Read the model definition and answer for the solid it produces. Units are mm, in the model's axes. A direction names the side the tool comes from. Coordinates: 2 decimals unless noted, no trailing zeros. Loops run counter-clockwise (first coordinate to the right, second up) from the corner with the lowest first, then second, coordinate; pieces in that order, holes last. Notation, with made-up numbers: (62.5, -8) -> (67.5, -8) arc R35 cw to (67.5, 24) -> close; hole circle Ø2 at (22, 81.25). An arc over 180 degrees is marked (long way). Answer as a JSON object with one key per item and string values. Group by question number.
Q1. The part is cut by section C-C on x = -368. Write down the section's boundary in (y, z), and give its area (3 significant figures).
Q2. Each of these flat-tipped pins is pushed along its axis until it touches: P1, Ø2, axis at x = -12.5, y = 1.5, coming from the -Z side; P2, Ø6, axis at x = -262, z = 110.5, coming from the -Y side; P3, Ø12, axis at x = -310, y = -23, coming from the +Z side; P4, Ø2, axis at y = -34.5, z = 35.5, coming from the -X side. Where does it stop, or does it pass through?
Q3. The part is cut by section B-B on x = -136. Write down the section's boundary in (y, z), and give its area (3 significant figures).
Q4. Determine the mould class of faces 1 (the cylindrical face through (396.261, -12.828, -5.883)), 2 (the flat face through (321.003, -19, -14)), 3 (the flat face through (-258, -9.876, 54)) for opening direction Z: released by +Z, released by -Z, zero draft, split by the parting line, or undercut.
Q5. For faces 4 (the flat face through (-217.761, -25, 54)), 5 (the flat face through (-321.003, -14, -7)), 6 (the flat face through (-258, -40.692, 54)), determine the directions among +Z, -Z, +X, -X, +Y, -Y from which every point of the face is accessible in a straight line to the end or side of a thin tool.
Q6. Straight lines are drawn through the part: line 1 along Z through (x, y) = (313, -17.5); line 2 along X through (y, z) = (11, 110); line 3 along Y through (x, z) = (-270, -22). For each, find the intervals that lie inside material, in ascending order. Write a range as [from, to].
Q7. The part is cut by section A-A on z = 0. Write down the section's boundary in (x, y).
from build123d import *

# Parameters (mm, degrees)
F0_W      = 642.00504
F0_H      = 59.35203
F1_DEPTH  = 50.8
F2_R      = 13.138682
F3_DEPTH  = 181.356
F4_R      = 15.361359
F5_DEPTH  = 152.654
F6_W      = 78.62696
F6_H      = 30.816156
F7_DEPTH  = 48.514
F9_R      = 16.886995
F10_DEPTH = 101.6


with BuildPart() as f1:
    # F0 (on Front) → F1 (new body)
    with BuildSketch(Plane.XZ):
        Rectangle(F0_W, F0_H)
    extrude(amount=F1_DEPTH)

    # F2 (on face) → F3 (join)
    with BuildSketch(Plane(origin=(-321.00252, 0, 0), x_dir=(0, -1, 0), z_dir=(-1, 0, 0))):
        with Locations((26.228841, 0)):
            Circle(F2_R)
    extrude(amount=F3_DEPTH)

    # F4 (on face) → F5 (join)
    with BuildSketch(Plane.YZ.offset(321.00252)):
        with Locations((-27.018422, 0)):
            Circle(F4_R)
    extrude(amount=F5_DEPTH)

    # F6 (on face) → F7 (join)
    with BuildSketch(Plane.XY.offset(29.676015)):
        with Locations((-257.074803, -25.283979)):
            Rectangle(F6_W, F6_H)
    extrude(amount=F7_DEPTH)

    # F9 (on face) → F10 (join)
    with BuildSketch(Plane(origin=(0, 18.748979, 18.748979), x_dir=(1, 0, 0), z_dir=(0, -0.707107, -0.707107))):
        with Locations((-255.314887, 70.006117)):
            Circle(F9_R)
    extrude(amount=-F10_DEPTH)


solid = f1.part
Final values:
{
 "1": {"outline": "circle Ø26.28 at (-26.23, 0)", "area": "542 mm2"},
 "2": {"P1": "passes through", "P2": "stops at y = -13.84", "P3": "stops at z = 29.68", "P4": "stops at x = -296.39"},
 "3": {"outline": "(-50.8, -29.68) -> (0, -29.68) -> (0, 29.68) -> (-50.8, 29.68) -> close", "area": "3,020 mm2"},
 "4": {"face 1": "split by the parting line", "face 2": "zero draft", "face 3": "undercut"},
 "5": {"face 4": "+Z, +X, +Y, -Y", "face 5": "-X", "face 6": "+X, -X, -Y"},
 "6": {"line 1": "z = [-29.68, 29.68]", "line 2": "x = [-272.2, -238.43]", "line 3": "y = [-50.8, 0]"},
 "7": {"outline": "(-502.36, -39.37) -> (-321, -39.37) -> (-321, -50.8) -> (321, -50.8) -> (321, -42.38) -> (473.66, -42.38) -> (473.66, -11.66) -> (321, -11.66) -> (321, 0) -> (-321, 0) -> (-321, -13.09) -> (-502.36, -13.09) -> close"}
}
